Verification items for this drawing (mm, ordinates from the low corner). Round coordinates to 2 decimals unless told otherwise and drop trailing zeros. Loops run counter-clockwise (first coordinate to the right, second up) from the corner with the lowest first, then second, coordinate; pieces in that order, holes last. Notation, with made-up numbers: M 3,9.25 L 49,9.25 A25 ccw 49,35.25 Z; hole C 46.5,-24 d3. An arc over 180 degrees is marked long. One line per item, written item: value.
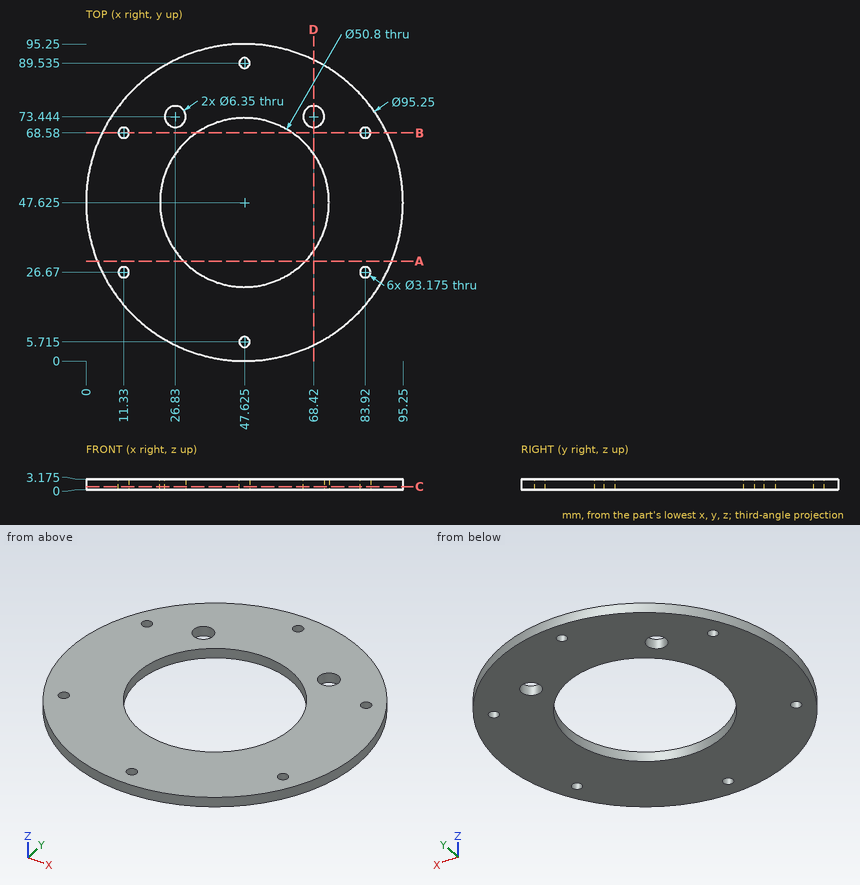
(1) Thickness scan on L1, parallel to Y at x = 69.5, z = 1.5; L2, parallel to X at y = 68.58, z = 1.2; L3, parallel to Y at x = 24.5, z = 1.9. Record the ranges inside material, lowest first. Write a range as from..to.
Completed:
L1: y = 5.32..34.72, 60.53..70.46, 76.43..89.93
L2: x = 4.86..9.74, 12.92..33.27, 61.98..82.33, 85.51..90.39
L3: y = 5.99..37.12, 58.13..71.29, 75.6..89.26
(2) Sectioned sample at C-C on z = 0.85. Count the separate pieces of the cut face and the enclosed holes in it, and give its area (3 significant figures).
Completed:
separate pieces: 1
enclosed holes: 9
area: 4,990 mm^2
(3) Sectioned sample at B-B on y = 68.58. Enter the section's corners in (x, z) (1 decimal).
Completed:
outline: M 4.9,0 L 9.7,0 L 9.7,3.2 L 4.9,3.2 Z; M 12.9,0 L 33.3,0 L 33.3,3.2 L 12.9,3.2 Z; M 62,0 L 82.3,0 L 82.3,3.2 L 62,3.2 Z; M 85.5,0 L 90.4,0 L 90.4,3.2 L 85.5,3.2 Z
(4) Sectioned sample at A-A on y = 30. Enter the section's corners in (x, z) (1 decimal).
Completed:
outline: M 3.4,0 L 29.3,0 L 29.3,3.2 L 3.4,3.2 Z; M 65.9,0 L 91.9,0 L 91.9,3.2 L 65.9,3.2 Z
(5) Sectioned sample at D-D on x = 68.42. Enter the section's corners in (y, z) (3 decimals), and give its area (3 significant figures).
Completed:
outline: M 4.78,0 L 33.04,0 L 33.04,3.175 L 4.78,3.175 Z; M 62.21,0 L 70.269,0 L 70.269,3.175 L 62.21,3.175 Z; M 76.619,0 L 90.47,0 L 90.47,3.175 L 76.619,3.175 Z
area: 159 mm^2
(6) Depth check by flat-ended pin: pin 1 Ø1 at (x, z) = (79.5, 1.5) entering from +Y. Enter the tip coordinate at first touch or a pass-through.
Completed:
pin 1: stops at y = 83.45
